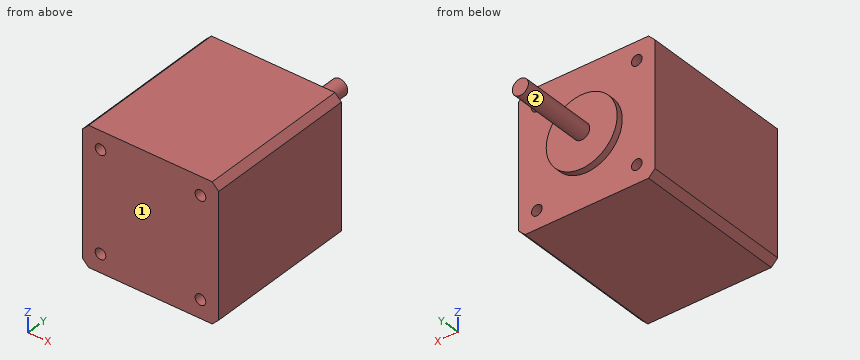
Autodesk Inventor part; units mm, degrees
ref_plane "YZ Plane" through (0, 0, 0) normal (1, 0, 0) x (0, 1, 0)
ref_plane "XZ Plane" through (0, 0, 0) normal (0, 1, 0) x (-1, 0, 0)
ref_plane "XY Plane" through (0, 0, 0) normal (0, 0, 1) x (1, 0, 0)
sketch "Sketch1" plane through (0, 0, 0) normal (0, 1, 0) x (-1, 0, 0)
  line L0 (19.15, -21.15) -> (-19.15, -21.15)
  line L1 (-21.15, -19.15) -> (-21.15, 19.15)
  line L2 (-19.15, 21.15) -> (19.15, 21.15)
  line L3 (21.15, 19.15) -> (21.15, -19.15)
  line L4 (21.15, -21.15) -> (-21.15, 21.15) construction
  line L5 (-21.15, -21.15) -> (21.15, 21.15) construction
  line L6 (-19.15, 21.15) -> (-21.15, 19.15)
  line L7 (-19.15, -21.15) -> (-21.15, -19.15)
  line L8 (19.15, -21.15) -> (21.15, -19.15)
  line L9 (19.15, 21.15) -> (21.15, 19.15)
  point P0 (0, 0)
  dimension "d0" = 42.3
  dimension "d1" = 42.3
  dimension "d2" = 2
  dimension "d3" = 2
  dimension "d4" = 2
  dimension "d5" = 2
  dimension "d6" = 2
  dimension "d7" = 2
  dimension "d8" = 2
  dimension "d9" = 2
extrude "Extrusion1" add sketch "Sketch1" along normal blind 48
sketch "Sketch3" plane through (0, 48, 0) normal (0, 1, 0) x (1, 0, 0)
  line L0 (15.5, -15.5) -> (-15.5, -15.5)
  line L1 (-15.5, -15.5) -> (-15.5, 15.5)
  line L2 (-15.5, 15.5) -> (15.5, 15.5)
  line L3 (15.5, 15.5) -> (15.5, -15.5)
  line L4 (15.5, -15.5) -> (-15.5, 15.5) construction
  line L5 (-15.5, -15.5) -> (15.5, 15.5) construction
  circle A0 centre (-15.5, 15.5) radius 1.65
  circle A1 centre (15.5, 15.5) radius 1.65
  circle A2 centre (-15.5, -15.5) radius 1.65
  circle A3 centre (15.5, -15.5) radius 1.65
  point P0 (0, 0)
  dimension "d15" = 31
  dimension "d16" = 31
  dimension "d17" = 3.3
  dimension "d18" = 3.3
  dimension "d19" = 3.3
  dimension "d20" = 3.3
hole "Hole1" at (15.5, 48, -15.5) at (15.5, 48, 15.5) at (-15.5, 48, 15.5) at (-15.5, 48, -15.5) direction (0, -1, 0) diameter 3.3 end through all
sketch "Sketch2" plane through (0, 48, 0) normal (0, 1, 0) x (1, 0, 0)
  circle A0 centre (0, 0) radius 11
  dimension "d12" = 22
extrude "Extrusion2" add sketch "Sketch2" along normal blind 2
sketch "Sketch4" plane through (0, 50, 0) normal (0, 1, 0) x (1, 0, 0)
  circle A0 centre (0, 0) radius 11
  circle A1 centre (0, 0) radius 2.5
  dimension "d28" = 5
extrude "Extrusion3" add sketch "Sketch4" along normal blind 24 contours A1
equation "\"d3\" = d2"
equation "\"d4\" = d2"
equation "\"d5\" = d4"
equation "\"d6\" = d2"
equation "\"d7\" = d6"
equation "\"d8\" = d2"
equation "\"d9\" = d8"
properties part number "nema17"
Verification items for the finished model (mm, model axes). Face numbers are marked on the shaded views. A direction names the side the tool comes from. Give positions to 0.01 mm unless a question says otherwise; leave off trailing zeros. Order: outer loops, then holes, each group sorted by start corner. A loop starts at its lowest first (then second) coordinate and runs counter-clockwise, first axis right, second up. Notation, with made-up numbers: (76, -27) - (100, -27) arc R16 cw to (100, -8) - close; hole circle Ø10 at (77.5, 0). An arc over 180 degrees is marked (long way). Answer as CSV lines item,"result". Start each with the question number.
Item 1: Section check C-C, the plane y = 26. Record the boundary of the cut face in (x, z).
Item 2: Section check A-A, the plane x = 15.5. Record the boundary of the cut face in (y, z).
Item 3: Access from +Z, -Z, +X, -X, +Y, -Y to the whole of each face (thin tool, end or side, straight path). Record for the marked faces 1 and 2.
Item 4: Material ranges on L1, parallel to X at y = 16, z = -15.5; L2, parallel to Z at x = 16.5, y = 33, recorded low to high.
Item 5: Gauge pin test, flat ends, axial feed: pin 1 (3 mm diameter, centred on x = -15, z = -2.5, fed in from -Y); pin 2 (5.5 mm diameter, centred on x = 15.5, z = 15.5, fed in from +Y). Record the tip position at first contact, or that the pin passes through.
Item 6: Section check B-B, the plane z = 15.5. Record the boundary of the cut face in (x, y), plus the area to 3 significant figures.
Item 7: Section check D-D, the plane x = 0. Record the boundary of the cut face in (y, z), plus the area to 3 significant figures.
Filled in:
1,outline,"(-21.15, -19.15) - (-19.15, -21.15) - (19.15, -21.15) - (21.15, -19.15) - (21.15, 19.15) - (19.15, 21.15) - (-19.15, 21.15) - (-21.15, 19.15) - close; hole circle Ø3.3 at (-15.5, -15.5); hole circle Ø3.3 at (-15.5, 15.5); hole circle Ø3.3 at (15.5, -15.5); hole circle Ø3.3 at (15.5, 15.5)"
2,outline,"(0, -21.15) - (48, -21.15) - (48, -17.15) - (0, -17.15) - close; (0, -13.85) - (48, -13.85) - (48, 13.85) - (0, 13.85) - close; (0, 17.15) - (48, 17.15) - (48, 21.15) - (0, 21.15) - close"
3,face 1,"+Z, -Z, +X, -X, -Y"
3,face 2,"+Y"
4,L1,"-21.15 to -17.15, -13.85 to 13.85, 17.15 to 21.15"
4,L2,"-21.15 to -16.81, -14.19 to 14.19, 16.81 to 21.15"
5,pin 1,"y = 0"
5,pin 2,"y = 48"
6,outline,"(-21.15, 0) - (-17.15, 0) - (-17.15, 48) - (-21.15, 48) - close; (-13.85, 0) - (13.85, 0) - (13.85, 48) - (-13.85, 48) - close; (17.15, 0) - (21.15, 0) - (21.15, 48) - (17.15, 48) - close"
6,area,"1,710 mm^2"
7,outline,"(0, -21.15) - (48, -21.15) - (48, -11) - (50, -11) - (50, -2.5) - (74, -2.5) - (74, 2.5) - (50, 2.5) - (50, 11) - (48, 11) - (48, 21.15) - (0, 21.15) - close"
7,area,"2,190 mm^2"
